Geometry check sheet. Reference: the model listing, model coordinates, mm. A direction names the side the tool comes from. Coordinates: 2 decimals unless noted, no trailing zeros. Write each loop counter-clockwise with the first axis right and the second up, starting at its lowest first coordinate (ties: lowest second). Pieces come first, ordered by that corner, then holes. Notation, with made-up numbers: M 26,-35.75 L 68,-35.75 A32 cw 68,-0.75 Z; hole C 53,44.25 d10. An arc over 180 degrees is marked long. Put each result on its own line as item: value. Start each with the question number.
1) Gauge pin test, flat ends, axial feed: pin 1 (6 mm diameter, centred on y = 152.4, z = 0, fed in from -X); pin 2 (12 mm diameter, centred on y = 3.5, z = -7.5, fed in from +X); pin 3 (1 mm diameter, centred on y = -1.5, z = 21.5, fed in from -X); pin 4 (12 mm diameter, centred on x = -15, z = -19.5, fed in from -Y). Record the tip position at first contact, or that the pin passes through.
2) Cross-section at B-B on z = 0. Record the cut outline in (x, y), plus the area to 3 significant figures.
3) Cross-section at D-D on y = 109. Record the cut outline in (x, z).
4) Cross-section at A-A on x = 0. Record the cut outline in (y, z), plus the area to 3 significant figures.
5) Set-up check for faces 1 (the cylindrical face through (34.446, 152.295, -2.498)), 2 (the flat face through (-28, -30, -18)), 3 (the flat face through (29, 0, 18)), 4 (the cylindrical face through (-21, 99, -28)), 5 (the cylindrical face through (33.71, 99.61, -4.43)): record each of +Z, -Z, +X, -X, +Y, -Y from which the full face is reachable in a straight line by a thin tool's end or side.
6) Scan lines: line 1 along X through (y, z) = (144, 1); line 2 along Z through (x, y) = (9, 74.5); line 3 along Z through (x, y) = (10, 144.5). Record each from-to range of solid material in increasing order.
7) Cross-section at C-C on z = -20. Record the cut outline in (x, y).
8) Mould release check, pull along X, two halves, no side actions. Record for faces 6 (the flat face through (28, 2, 18)), 7 (the flat face through (34, 200, -5)), 8 (the cylindrical face through (-33.61, -15.21, -4.41)), 9 (the cylindrical face through (-32.12, -14.22, 7.13)): released by +X, released by -X, zero draft, split by the parting line, or undercut.
from build123d import *

# Parameters (mm, degrees)
SKETCH1_R           = 35
SKETCH1_R_2         = 34
BOSS_EXTRUDE1_DEPTH = 200
SKETCH2_R           = 34
SKETCH2_R_2         = 32.9
BOSS_EXTRUDE2_DEPTH = 2
BOSS_EXTRUDE3_START = 30
SKETCH3_R           = 33.9
SKETCH3_R_2         = 32.9
BOSS_EXTRUDE3_DEPTH = 30
SKETCH4_R           = 2.5
CUT_EXTRUDE1_DEPTH  = 40


with BuildPart() as part:
    # Sketch1 → Boss-Extrude1 (new body)
    with BuildSketch(Plane(origin=(0, 0, 0), x_dir=(1, 0, 0), z_dir=(0, 1, 0))):
        with Locations(Location((0, 0, 0), (0, 0, 270))):
            Circle(SKETCH1_R)
        with Locations(Location((0, 0, 0), (0, 0, 270))):
            Circle(SKETCH1_R_2, mode=Mode.SUBTRACT)
    extrude(amount=BOSS_EXTRUDE1_DEPTH)

    # Sketch2 → Boss-Extrude2 (add)
    with BuildSketch(Plane.XZ):
        with Locations(Location((0, 0, 0), (0, 0, 270))):
            Circle(SKETCH2_R)
        with Locations(Location((0, 0, 0), (0, 0, 270))):
            Circle(SKETCH2_R_2, mode=Mode.SUBTRACT)
    extrude(amount=-BOSS_EXTRUDE2_DEPTH)

    # Sketch3 → Boss-Extrude3 (add)
    with BuildSketch(Plane.XZ.offset(BOSS_EXTRUDE3_START)):
        with Locations(Location((0, 0, 0), (0, 0, 90))):
            Circle(SKETCH3_R)
        with Locations(Location((0, 0, 0), (0, 0, 270))):
            Circle(SKETCH3_R_2, mode=Mode.SUBTRACT)
    extrude(amount=-BOSS_EXTRUDE3_DEPTH)

    # Sketch4 → Cut-Extrude1 (cut)
    with BuildSketch(Plane(origin=(0, 0, 0), x_dir=(0, 0, -1), z_dir=(1, 0, 0))):
        with Locations(Location((0, 152.404493748, 0), (0, 0, 180))):
            Circle(SKETCH4_R)
    extrude(amount=CUT_EXTRUDE1_DEPTH, mode=Mode.SUBTRACT)


solid = part.part
Answer key:
1. pin 1: stops at x = -35
1. pin 2: stops at x = 34.97
1. pin 3: stops at x = -26.61
1. pin 4: passes through
2. outline: M -35,0 L -33.9,0 L -33.9,-30 L -32.9,-30 L -32.9,2 L -34,2 L -34,200 L -35,200 Z; M 32.9,-30 L 33.9,-30 L 33.9,0 L 35,0 L 35,149.9 L 34,149.9 L 34,2 L 32.9,2 Z; M 34,154.9 L 35,154.9 L 35,200 L 34,200 Z
2. area: 459 mm²
3. outline: C 0,0 d70; hole C 0,0 d68
4. outline: M -30,-33.9 L 0,-33.9 L 0,-35 L 200,-35 L 200,-34 L 2,-34 L 2,-32.9 L -30,-32.9 Z; M -30,32.9 L 2,32.9 L 2,34 L 200,34 L 200,35 L 0,35 L 0,33.9 L -30,33.9 Z
4. area: 464 mm²
5. face 1: +X
5. face 2: +Z, -Z, +X, -X, -Y
5. face 3: -Y
5. face 4: +Y, -Y
5. face 5: +Y
6. line 1: x = -34.99 to -33.99, 33.99 to 34.99
6. line 2: z = -33.82 to -32.79, 32.79 to 33.82
6. line 3: z = -33.54 to -32.5, 32.5 to 33.54
7. outline: M -28.72,0 L -27.37,0 L -27.37,-30 L -26.12,-30 L -26.12,2 L -27.5,2 L -27.5,200 L -28.72,200 Z; M 26.12,-30 L 27.37,-30 L 27.37,0 L 28.72,0 L 28.72,200 L 27.5,200 L 27.5,2 L 26.12,2 Z
8. face 6: undercut
8. face 7: zero draft
8. face 8: split by the parting line
8. face 9: undercut
